Work out the finished part from the listing and answer in its coordinate system (mm). A direction names the side the tool comes from. Give positions to 0.01 mm unless a question says otherwise; leave off trailing zeros. Loops run counter-clockwise (first coordinate to the right, second up) from the corner with the lowest first, then second, coordinate; pieces in that order, holes last. Notation, with made-up numbers: (8, 13) - (12, 13) arc R23 ccw to (12, 50) - close; hole circle Ø10 at (16, -26.5). An arc over 180 degrees is marked (long way). Use CSV: the item, a comma, the result in double quotes.
Autodesk Inventor part; units mm, degrees
ref_plane "YZ Plane" through (0, 0, 0) normal (1, 0, 0) x (0, 1, 0)
ref_plane "XZ Plane" through (0, 0, 0) normal (0, 1, 0) x (-1, 0, 0)
ref_plane "XY Plane" through (0, 0, 0) normal (0, 0, 1) x (1, 0, 0)
sketch "スケッチ1" plane through (0, 0, 0) normal (0, 1, 0) x (-1, 0, 0)
  line L0 (0, 0) -> (-90, 0)
  line L1 (-90, 0) -> (-90, 10)
  line L2 (-90, 10) -> (0, 10)
  line L3 (0, 10) -> (0, 0)
  dimension "d0" = 90
  dimension "d1" = 10
extrude "押し出し1" add sketch "スケッチ1" along normal blind 0.5
sketch "スケッチ2" plane through (0, 0, 0) normal (-1, 0, 0) x (0, 0, 1)
  line L0 (10, 0) -> (0, 0)
  line L1 (10, 0) -> (10, 0.5)
  line L2 (0, 0.5) -> (10, 0.5)
  line L3 (0, 0) -> (0, 0.5)
  line L4 (0, 0) -> (10, 0)
  line L5 (10, 0) -> (10, 5)
  line L6 (10, 5) -> (0, 5)
  line L7 (0, 5) -> (0, 0)
  dimension "d4" = 5
extrude "押し出し2" add sketch "スケッチ2" along normal blind 5 contours L2 L7 L6 L5
sketch "スケッチ3" plane through (0, 0, 0) normal (-1, 0, 0) x (0, 0, 1)
  line L0 (10, 0) -> (0, 0)
  line L1 (10, 0) -> (10, 0.5)
  line L2 (0, 0.5) -> (10, 0.5)
  line L3 (0, 0) -> (0, 0.5)
extrude "押し出し3" add sketch "スケッチ3" along normal blind 5
sketch "スケッチ4" plane through (90, 0, 10) normal (1, 0, 0) x (0, 0, -1)
  line L0 (0, 0) -> (10, 0)
  line L1 (10, 0) -> (10, 5.0408)
  line L2 (10, 5.0408) -> (0, 5.0408)
  line L3 (0, 5.0408) -> (0, 0)
extrude "押し出し4" add sketch "スケッチ4" along normal blind 5
sketch "スケッチ5" plane through (0, 0.5, 0) normal (0, 0, -1) x (-1, 0, 0)
  line L0 (5, -0.5) -> (-95, -0.5)
  line L1 (5, 4.5) -> (5, -0.5)
  line L2 (0, 4.5) -> (5, 4.5)
  line L3 (0, 4.5) -> (0, 0)
  line L4 (-90, 0) -> (0, 0)
  line L5 (-90, 0) -> (-90, 4.5408)
  line L6 (-90, 4.5408) -> (-95, 4.5408)
  line L7 (-95, -0.5) -> (-95, 4.5408)
  line L8 (-95, -0.5) -> (5, -0.5)
  line L9 (5, -0.5) -> (5, 4.5)
  line L10 (5, 4.5) -> (-95, 4.5)
  line L11 (-95, 4.5) -> (-95, -0.5)
  point P0 (0, -0.5)
extrude "押し出し5" add sketch "スケッチ5" along normal blind 2
sketch "スケッチ6" plane through (0, 0.5, 10) normal (0, 0, 1) x (1, 0, 0)
  line L0 (95, -0.5) -> (-5, -0.5)
  line L1 (95, 4.5408) -> (95, -0.5)
  line L2 (-5, -0.5) -> (95, -0.5)
  line L3 (95, -0.5) -> (95, 4.5408)
  line L4 (95, 4.5408) -> (-5, 4.5408)
  line L5 (-5, 4.5408) -> (-5, -0.5)
  point P0 (0, -0.5)
extrude "押し出し6" add sketch "スケッチ6" along normal blind 2
sketch "スケッチ7" plane through (90, 5.0408, -2) normal (0, 1, 0) x (1, 0, 0)
  line L0 (0, -12) -> (0, 0)
  line L1 (0, -12) -> (-95, -12)
  line L2 (-95, -12) -> (-95, -14)
  line L3 (5, -14) -> (-95, -14)
  line L4 (5, -14) -> (5, 0)
  line L5 (0, 0) -> (5, 0)
  point P0 (-90, -2)
sketch "スケッチ8" plane through (0, 0.5, 12) normal (0, 0, 1) x (1, 0, 0)
  line L0 (95, 4.5408) -> (-5, 4.5408)
  line L1 (27.5, 9.1315) -> (62.5, 9.1315)
  line L2 (62.5, 9.1315) -> (62.5, -0.0498)
  line L3 (62.5, -0.0498) -> (27.5, -0.0498)
  line L4 (27.5, -0.0498) -> (27.5, 9.1315)
  line L5 (27.5, 9.1315) -> (62.5, -0.0498) construction
  line L6 (62.5, 9.1315) -> (27.5, -0.0498) construction
  point P0 (0, -0.5)
  point P1 (45, 4.5408)
  dimension "d15" = 35
extrude "押し出し7" cut sketch "スケッチ8" against normal blind 20
properties part number "知能ロボコン砲台スペーサ高さ"
Item 1: For faces 1 (the flat face through (44.3, 0.3, 12)), 2 (the flat face through (45, 0.45, 5)), 3 (the flat face through (0, 3, 5)), determine the directions among +Z, -Z, +X, -X, +Y, -Y from which every point of the face is accessible in a straight line to the end or side of a thin tool.
Determined:
face 1,"+Z, +X, -X, +Y, -Y"
face 2,"+Z, -Z, +Y"
face 3,"+Y"
Item 2: A cutting plane is placed at A-A on y = 3.5. Determine the outline of the cut face in (x, z).
Determined:
outline,"(-5, -2) - (27.5, -2) - (27.5, 0) - (0, 0) - (0, 10) - (27.5, 10) - (27.5, 12) - (-5, 12) - close; (62.5, -2) - (95, -2) - (95, 12) - (62.5, 12) - (62.5, 10) - (90, 10) - (90, 0) - (62.5, 0) - close"
Item 3: The mould has two halves that part along Z. Classify faces 4 (the flat face through (11, 5.041, 11)), 5 (the flat face through (45.7, 0.3, -2)), 6 (the flat face through (76, 3, 0)): pulls with the +Z half, pulls with the -Z half, needs draft (parallel to the pull), parting line crosses it, or undercut.
Determined:
face 4,"needs draft"
face 5,"pulls with the -Z half"
face 6,"undercut"
Item 4: A cutting plane is placed at B-B on z = -1. Determine the outline of the cut face in (x, y), and give its area (3 significant figures).
Determined:
outline,"(-5, 0) - (95, 0) - (95, 5.04) - (90, 5.04) - (90, 5) - (62.5, 5) - (62.5, 0.45) - (27.5, 0.45) - (27.5, 5) - (-5, 5) - close"
area,"341 mm²"
Item 5: A cutting plane is placed at D-D on z = 5. Determine the outline of the cut face in (x, y), and give its area (3 significant figures).
Determined:
outline,"(-5, 0) - (95, 0) - (95, 5.04) - (90, 5.04) - (90, 0.5) - (62.5, 0.5) - (62.5, 0.45) - (27.5, 0.45) - (27.5, 0.5) - (0, 0.5) - (0, 5) - (-5, 5) - close"
area,"93.5 mm²"
Item 6: Given P1, Ø1.6, axis at x = 75.5, z = -1, coming from the +Y side; P2, Ø3, axis at x = 77.5, z = 2.5, coming from the +Y side, each flat-ended and moving along its own axis, determine where each tip first touches the part or whether it passes through.
Determined:
P1,"stops at y = 5"
P2,"stops at y = 0.5"
Item 7: A cutting plane is placed at C-C on x = 20. Determine the outline of the cut face in (y, z).
Determined:
outline,"(0, -2) - (5, -2) - (5, 0) - (0.5, 0) - (0.5, 10) - (5.04, 10) - (5.04, 12) - (0, 12) - close"
Item 8: Find the intervals of material crossed by line 1 (X direction, y = 2.05, z = 10.5); line 2 (Z direction, x = 0.5, y = 3.45); line 3 (X direction, y = 2.8, z = 8.25), in increasing order.
Determined:
line 1,"x = -5 to 27.5, 62.5 to 95"
line 2,"z = -2 to 0, 10 to 12"
line 3,"x = -5 to 0, 90 to 95"
